Part model, mm, in its own coordinate system. Round coordinates to 2 decimals unless told otherwise and drop trailing zeros. Loops run counter-clockwise (first coordinate to the right, second up) from the corner with the lowest first, then second, coordinate; pieces in that order, holes last.
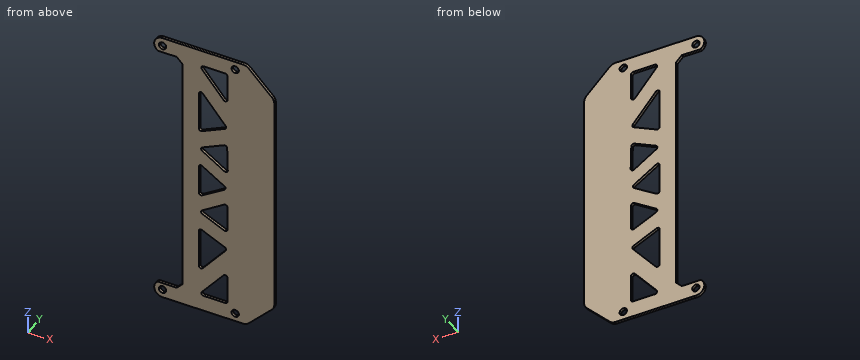
Autodesk Inventor part; units mm, degrees
ref_plane "YZ Plane" through (0, 0, 0) normal (1, 0, 0) x (0, 1, 0)
ref_plane "XZ Plane" through (0, 0, 0) normal (0, 1, 0) x (-1, 0, 0)
ref_plane "XY Plane" through (0, 0, 0) normal (0, 0, 1) x (1, 0, 0)
sketch "Sketch1" plane through (0, 0, 0) normal (0, 1, 0) x (-1, 0, 0)
  circle A0 centre (0, 0) radius 2.0955
  circle A1 centre (41.2753, 0) radius 2.0955
  circle A2 centre (0, -150.8125) radius 2.0955
  circle A3 centre (41.2753, -150.8125) radius 2.0955
  arc A4 (43.9079, -3.9688) -> (41.2753, 4.7625) centre (41.2753, 0) ccw
  arc A5 (41.2753, -155.575) -> (43.9079, -146.8438) centre (41.2753, -150.8125) ccw
  line L0 (29.8453, -7.366) -> (29.8453, -143.4465)
  line L1 (41.2753, -155.575) -> (0, -155.575)
  line L2 (0, 4.7625) -> (41.2753, 4.7625)
  line L3 (33.2426, -3.9688) -> (29.8453, -7.366)
  line L4 (29.8453, -143.4465) -> (33.2426, -146.8438)
  line L5 (17.9778, -146.431) -> (5.6515, -146.431)
  line L6 (5.6515, -4.3815) -> (17.9778, -4.3815)
  line L7 (18.9507, -6.4678) -> (6.6244, -21.1577)
  line L8 (20.7013, -4.3815) -> (39.8776, -4.3815) construction
  line L9 (18.4584, -21.28) -> (5.4454, -36.7883)
  line L10 (5.8815, -38.7557) -> (18.8946, -44.8238)
  line L11 (4.3815, -38.0562) -> (18.7398, -38.0562) construction
  line L12 (18.6151, -54.7828) -> (6.3567, -49.0665)
  line L13 (6.1698, -65.111) -> (18.7659, -57.0016)
  line L14 (18.9507, -144.3447) -> (6.6244, -129.6548)
  line L15 (20.7013, -146.431) -> (39.8776, -146.431) construction
  line L16 (18.4584, -129.5325) -> (5.4454, -114.0242)
  line L17 (5.8815, -112.0568) -> (18.8946, -105.9887)
  line L18 (4.3815, -112.7563) -> (18.7398, -112.7563) construction
  line L19 (18.6151, -96.0297) -> (6.1882, -101.8245)
  line L20 (18.7659, -93.8109) -> (6.339, -85.8105)
  line L21 (20.7013, -95.0569) -> (35.4808, -95.0569) construction
  line L22 (6.0792, -76.4797) -> (18.7526, -84.4929)
  line L23 (6.0792, -74.3328) -> (18.7526, -66.3196)
  line L24 (4.3815, -20.3414) -> (4.3815, -5.6515)
  line L25 (20.7013, -22.0963) -> (20.7013, -43.6728)
  line L26 (4.2127, -64.0121) -> (4.5503, -50.1866)
  line L27 (20.7013, -67.3931) -> (20.7013, -83.4194)
  line L28 (20.7013, -107.1397) -> (20.7013, -128.7162)
  line L29 (4.3815, -145.161) -> (4.3815, -130.4711)
  line L30 (4.3815, -100.6735) -> (4.3815, -86.8783)
  arc A6 (4.3815, -20.3414) -> (6.6244, -21.1577) centre (5.6515, -20.3414) ccw
  arc A7 (5.6515, -4.3815) -> (4.3815, -5.6515) centre (5.6515, -5.6515) ccw
  arc A8 (18.9507, -6.4678) -> (17.9778, -4.3815) centre (17.9778, -5.6515) ccw
  arc A9 (20.7013, -22.0963) -> (18.4584, -21.28) centre (19.4313, -22.0963) ccw
  arc A10 (5.4454, -36.7883) -> (5.8815, -38.7557) centre (6.4183, -37.6047) ccw
  arc A11 (18.8946, -44.8238) -> (20.7013, -43.6728) centre (19.4313, -43.6728) ccw
  arc A12 (6.3567, -49.0665) -> (4.5503, -50.1866) centre (5.8199, -50.2176) ccw
  arc A13 (4.2127, -64.0121) -> (6.1698, -65.111) centre (5.4823, -64.0431) ccw
  arc A14 (18.7659, -57.0016) -> (18.6151, -54.7828) centre (18.0784, -55.9338) ccw
  arc A15 (6.0792, -74.3328) -> (6.0792, -76.4797) centre (6.7579, -75.4063) ccw
  arc A16 (18.7526, -84.4929) -> (20.7013, -83.4194) centre (19.4313, -83.4194) ccw
  arc A17 (20.7013, -67.3931) -> (18.7526, -66.3196) centre (19.4313, -67.3931) ccw
  arc A18 (6.339, -85.8105) -> (4.3815, -86.8783) centre (5.6515, -86.8783) ccw
  arc A19 (18.6151, -96.0297) -> (18.7659, -93.8109) centre (18.0784, -94.8787) ccw
  arc A20 (4.3815, -100.6735) -> (6.1882, -101.8245) centre (5.6515, -100.6735) ccw
  arc A21 (20.7013, -107.1397) -> (18.8946, -105.9887) centre (19.4313, -107.1397) ccw
  arc A22 (5.8815, -112.0568) -> (5.4454, -114.0242) centre (6.4183, -113.2078) ccw
  arc A23 (18.4584, -129.5325) -> (20.7013, -128.7162) centre (19.4313, -128.7162) ccw
  arc A24 (6.6244, -129.6548) -> (4.3815, -130.4711) centre (5.6515, -130.4711) ccw
  arc A25 (4.3815, -145.161) -> (5.6515, -146.431) centre (5.6515, -145.161) ccw
  arc A26 (17.9778, -146.431) -> (18.9507, -144.3447) centre (17.9778, -145.161) ccw
  line L31 (0, 4.7625) -> (-4.3773, 4.7625)
  line L32 (-22.225, -13.0852) -> (-22.225, -137.7273)
  line L33 (-4.3773, -155.575) -> (0, -155.575)
  line L34 (43.9079, -3.9688) -> (33.2426, -3.9688)
  line L35 (43.9079, -146.8438) -> (33.2426, -146.8438)
  line L36 (-20.8301, -9.7176) -> (-7.7449, 3.3676)
  line L37 (-20.8301, -141.0949) -> (-7.7449, -154.1801)
  arc A27 (-4.3773, 4.7625) -> (-7.7449, 3.3676) centre (-4.3773, 0) ccw
  arc A28 (-20.8301, -9.7176) -> (-22.225, -13.0852) centre (-17.4625, -13.0852) ccw
  arc A29 (-22.225, -137.7273) -> (-20.8301, -141.0949) centre (-17.4625, -137.7273) ccw
  arc A30 (-7.7449, -154.1801) -> (-4.3773, -155.575) centre (-4.3773, -150.8125) ccw
  point P0 (29.8453, -4.7625)
  point P1 (29.8453, -146.05)
  point P2 (32.8298, -4.3815)
  point P3 (32.4488, -146.05)
  point P4 (-17.4625, 4.7625)
  point P5 (-22.225, 0)
  point P6 (-17.4625, -155.575)
  point P7 (-22.225, -150.8125)
  point P8 (-22.225, 4.7625)
  point P9 (-22.225, -11.1125)
  point P10 (-6.35, 4.7625)
  point P11 (-22.225, 4.7625)
  point P12 (-22.225, -139.7)
  point P13 (-6.35, -155.575)
  point P14 (-22.225, -155.575)
  point P15 (4.3815, -57.0993)
  dimension "d0" = 4.191
  dimension "d3" = 9.525
  dimension "d20" = 1.27
  dimension "d24" = 22.225
  dimension "d27" = 15.875
  dimension "d28" = 15.875
  dimension "d29" = 15.875
  dimension "d30" = 15.875
  dimension "d31" = 4.7625
extrude "Extrusion1" add sketch "Sketch1" along normal blind 1.5875
equation "\"BendRadius\" = Thickness"
equation "\"BendReliefWidth\" = Thickness"
equation "\"BendReliefDepth\" = 0.5 * Thickness"
equation "\"CornerReliefSize\" = 4 * Thickness"
equation "\"MinimumRemnant\" = 2 * Thickness"
equation "\"TransitionRadius\" = BendRadius"
equation "\"JacobiRadiusSize\" = BendRadius"
equation "\"GapSize\" = Thickness"
properties part number "ramp" material "Acetal Resin, White"
1) Slice it at A-A, the plane x = 0. Give the cut face in (y, z) (1 decimal).
Values:
outline: (0, -155.6) - (1.6, -155.6) - (1.6, -152.9) - (0, -152.9) - close; (0, -148.7) - (1.6, -148.7) - (1.6, -2.1) - (0, -2.1) - close; (0, 2.1) - (1.6, 2.1) - (1.6, 4.8) - (0, 4.8) - close
2) Slice it at B-B, the plane x = -35.5. Give the cut face in (y, z) (1 decimal).
Values:
outline: (0, -155.6) - (1.6, -155.6) - (1.6, -146.8) - (0, -146.8) - close; (0, -4) - (1.6, -4) - (1.6, 4.8) - (0, 4.8) - close
3) Slice it at C-C, the plane x = -13.5. Give the number of separate pieces and of enclosed holes in the cut face, then the cut area to 3 significant figures.
Values:
separate pieces: 8
enclosed holes: 0
area: 136 mm2
4) Slice it at D-D, the plane z = 0. Give the cut face in (x, y).
Values:
outline: (-46.04, 0) - (-43.37, 0) - (-43.37, 1.59) - (-46.04, 1.59) - close; (-39.18, 0) - (-2.1, 0) - (-2.1, 1.59) - (-39.18, 1.59) - close; (2.1, 0) - (11.11, 0) - (11.11, 1.59) - (2.1, 1.59) - close
5) Drop a flat-ended pin along its axis: pin 1 Ø0.8 at (y, z) = (0.5, -94.5) entering from -X. Give the stop position or say it passes through.
Values:
pin 1: stops at x = -29.85
6) Wall check: line 1 along Z through (x, y) = (0, 1.3) (1 decimal); line 2 along Z through (x, y) = (-19.5, 1) (1 decimal); line 3 along Z through (x, y) = (-43, 0.25). Give the ranges that are in metal, low to high.
Values:
line 1: z = -155.6 to -152.9, -148.7 to -2.1, 2.1 to 4.8
line 2: z = -155.6 to -130, -105.9 to -84.7, -66.1 to -44.9, -20.8 to 4.8
line 3: z = -155.25 to -152, -149.62 to -146.84, -3.97 to -1.19, 1.19 to 4.44
